Work out the finished part from the listing and answer in its coordinate system (mm). Face numbers are marked on the shaded views. A direction names the side the tool comes from. Coordinates: 2 decimals unless noted, no trailing zeros. Order: outer loops, then holes, each group sorted by start corner. A loop starts at its lowest first (then second) coordinate and runs counter-clockwise, first axis right, second up. Notation, with made-up numbers: (-23, -21) -> (6, -21) arc R20 cw to (6, -12) -> close; hole circle Ø11 at (76, 48.5). An arc over 180 degrees is marked (long way). Write item = value, one per line. Start each with the question number.
Q1. The part is cut by section A-A, the plane x = 606.5. Determine the outline of the cut face in (y, z).
Q2. Which of the six approach directions +Z, -Z, +X, -X, +Y, -Y give full straight-line access (tool end or side, diameter ignored) to the marked faces 1 and 2?
Q3. Flat-ended cylindrical pins translate along their axes: pin 1 (12 mm diameter, centred on y = 486.5, z = 76.5, fed in from -X); pin 2 (24 mm diameter, centred on y = 499, z = 59, fed in from -X); pin 3 (1 mm diameter, centred on x = 246, z = 89, fed in from -Y); pin 4 (8 mm diameter, centred on x = 828, z = 64.5, fed in from -Y). Find the tip coordinate at first contact, or state that the pin passes through.
Q4. The part is cut by section C-C, the plane z = 24. Determine the outline of the cut face in (x, y).
Q5. Straight lines are drawn through the part: L1, parallel to Z at x = 72, y = 259.5; L2, parallel to Y at x = 811.5, z = 66. For each, find the intervals that lie inside material, in ascending order. Write a range as from..to.
Autodesk Inventor part; units mm, degrees
ref_plane "YZ Plane" through (0, 0, 0) normal (1, 0, 0) x (0, 1, 0)
ref_plane "XZ Plane" through (0, 0, 0) normal (0, 1, 0) x (-1, 0, 0)
ref_plane "XY Plane" through (0, 0, 0) normal (0, 0, 1) x (1, 0, 0)
sketch "Sketch1" plane through (0, 0, 0) normal (0, 0, 1) x (1, 0, 0)
  line L0 (0, 0) -> (1050, 0) construction
  line L1 (1050, 0) -> (1050, 1050)
  line L2 (1050, 1050) -> (0, 1050)
  line L3 (0, 1050) -> (0, 0) construction
  line L4 (0, 260) -> (260, 0)
  line L5 (0, 260) -> (0, 1050)
  line L6 (260, 0) -> (1050, 0)
  dimension "profundidad" = 790
  dimension "d22" = 790
  dimension "d23" = 1050
extrude "Extrusion1" add sketch "Sketch1" along normal blind 50
fillet "Fillet1" radius 50 1 edges at (130, 130, 50)
sketch "Sketch3" plane through (1050, 0, 0) normal (0, -1, 0) x (1, 0, 0)
  line L0 (-1050, 0) -> (0, 0)
  line L1 (0, 0) -> (-20, 0)
  line L2 (-20, 0) -> (-20, 80)
  line L3 (0, 100) -> (0, 100)
  line L4 (0, 100) -> (0, 0)
  arc A0 (0, 100) -> (-20, 80) centre (0, 80) ccw
  point P0 (-20, 100)
  dimension "d9" = 20
  dimension "d10" = 100
  dimension "d11" = 20
extrude "Extrusion2" add sketch "Sketch3" against normal up to surface (1050 mm away)
sketch "Sketch4" plane through (0, 1050, 0) normal (-1, 0, 0) x (0, 0, 1)
  line L0 (0, 0) -> (100, 0)
  line L1 (100, -1050) -> (100, 0)
  line L2 (0, 0) -> (100, 0)
  line L3 (100, 0) -> (100, 0)
  line L4 (80, -20) -> (0, -20)
  line L5 (0, -20) -> (0, 0)
  arc A0 (80, -20) -> (100, 0) centre (80, 0) ccw
  point P0 (0, -1050)
  point P1 (100, -20)
  dimension "d14" = 20
  dimension "d15" = 20
extrude "Extrusion3" add sketch "Sketch4" against normal up to surface (1050 mm away)
properties part number "meson_esquinero"
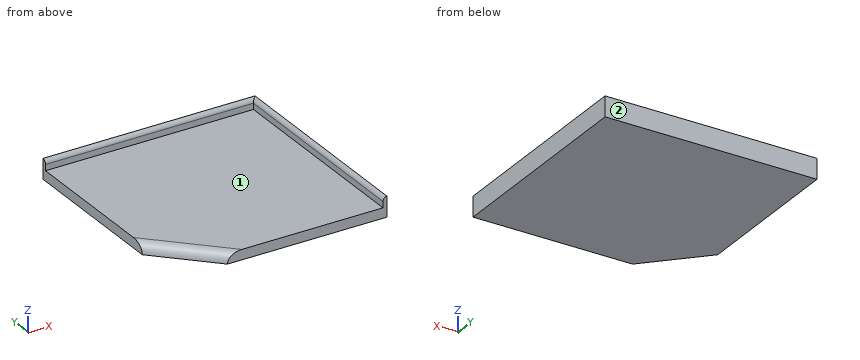
Model answer:
q1.outline = (0, 0) -> (1050, 0) -> (1050, 100) arc R20 ccw to (1030, 80) -> (1030, 50) -> (0, 50) -> close
q2.face_1 = +Z, -X, -Y
q2.face_2 = +Z, -Z, +X, -X, +Y
q3.pin_1 = 1030
q3.pin_2 = 0
q3.pin_3 = 1031.9
q3.pin_4 = 1030
q4.outline = (0, 268.68) -> (268.68, 0) -> (1050, 0) -> (1050, 1050) -> (0, 1050) -> close
q5.L1 = 0..50
q5.L2 = 1030..1050
